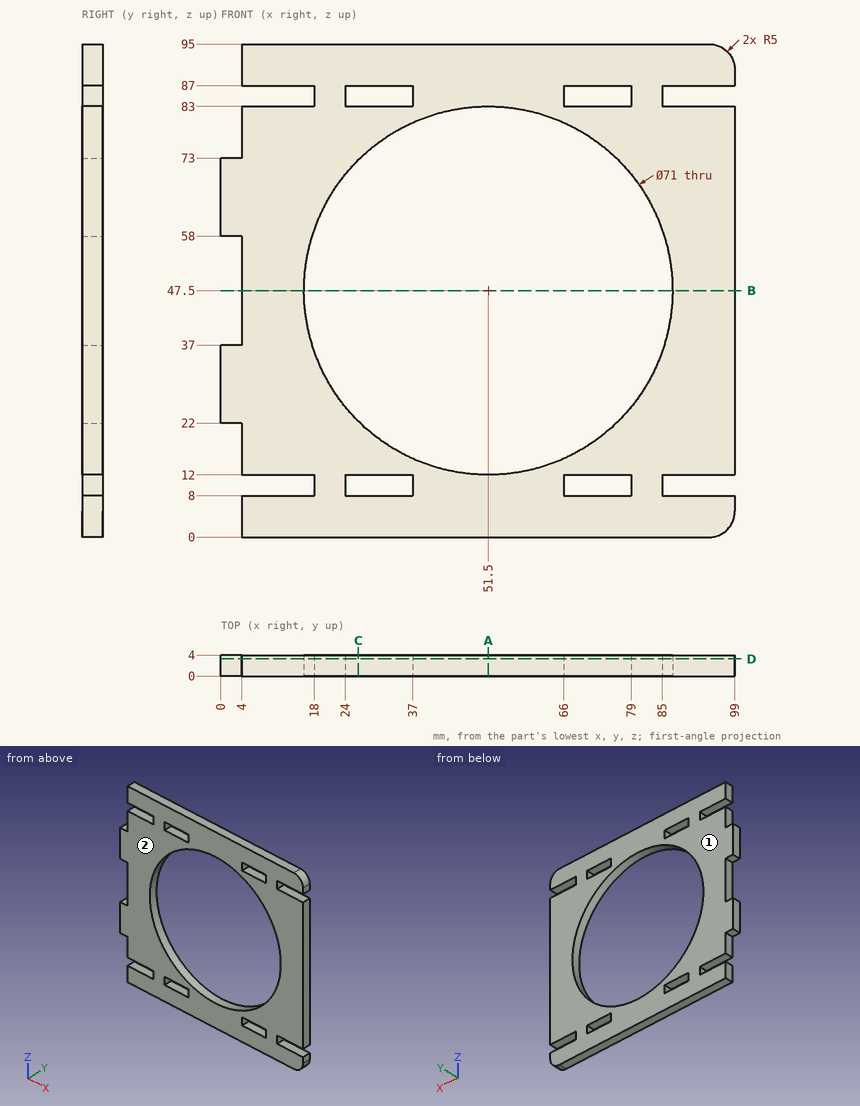
Part print with two shaded views. Sizes in mm from the minimum x, y, z corner. Coordinates: 2 decimals unless noted, no trailing zeros. Order: outer loops, then holes, each group sorted by start corner. A loop starts at its lowest first (then second) coordinate and runs counter-clockwise, first axis right, second up.
(1) Mould opens along Y. For the marked faces 1 and 2 say: released by +Y, released by -Y, zero draft, split by the parting line, or undercut.
Solution:
face 1: released by +Y
face 2: released by -Y
(2) Saw through at B-B, the plane z = 47.5. Write the cut outline in (x, y).
Solution:
outline: (4, 0) - (16, 0) - (16, 4) - (4, 4) - close; (87, 0) - (99, 0) - (99, 4) - (87, 4) - close
(3) Saw through at A-A, the plane x = 51.5. Write the cut outline in (y, z).
Solution:
outline: (0, 0) - (4, 0) - (4, 12) - (0, 12) - close; (0, 83) - (4, 83) - (4, 95) - (0, 95) - close
(4) Pin check, flat tips, straight feed: pin 1 Ø2 at (y, z) = (2, 85.5) entering from -X; pin 2 Ø2 at (x, y) = (2, 2.5) entering from +Z; pin 3 Ø1.2 at (y, z) = (2.5, 9.5) entering from +X. Stop position of each tip, or through.
Solution:
pin 1: stops at x = 18
pin 2: stops at z = 73
pin 3: stops at x = 85
(5) Saw through at C-C, the plane x = 26.5. Write the cut outline in (y, z).
Solution:
outline: (0, 0) - (4, 0) - (4, 8) - (0, 8) - close; (0, 12) - (4, 12) - (4, 22.3) - (0, 22.3) - close; (0, 72.7) - (4, 72.7) - (4, 83) - (0, 83) - close; (0, 87) - (4, 87) - (4, 95) - (0, 95) - close
(6) Saw through at D-D, the plane y = 3.3. Count the separate pieces of the cut face and the enclosed holes in it, and give its area (3 significant figures).
Solution:
separate pieces: 1
enclosed holes: 5
area: 4,740 mm2
(7) Drill centre lines: L1, parallel to X at y = 2.55, z = 47.5; L2, parallel to Z at x = 92, y = 0.3; L3, parallel to Z at x = 68, y = 0.6. Where is each one in solid material? Low to high.
Solution:
L1: x = 4 to 16, 87 to 99
L2: z = 0 to 8, 12 to 83, 87 to 95
L3: z = 0 to 8, 12 to 16.07, 78.93 to 83, 87 to 95
